```python
from build123d import *

# Parameters (mm, degrees)
SKETCH1_W           = 50.8
SKETCH1_H           = 61.92
BOSS_EXTRUDE2_DEPTH = 3.175
SKETCH2_R           = 12.5
SKETCH2_R_2         = 2.75
CUT_EXTRUDE1_DEPTH  = 4.175


with BuildPart() as part:
    # Sketch1 → Boss-Extrude2 (new body)
    with BuildSketch(Plane(origin=(0, 0, 0), x_dir=(0, 0, -1), z_dir=(1, 0, 0))):
        with Locations((25.4, 30.96)):
            Rectangle(SKETCH1_W, SKETCH1_H)
    extrude(amount=BOSS_EXTRUDE2_DEPTH)

    # Sketch2 → Cut-Extrude1 (cut, through all)
    with BuildSketch(Plane.ZY):
        with Locations((-25.399655405, 30.96)):
            Circle(SKETCH2_R)
        with Locations((-43.35992398, 48.920755906)):
            Circle(SKETCH2_R_2)
        with Locations((-25.399655405, 56.36)):
            Circle(SKETCH2_R_2)
        with Locations((-5.004504526, 56.648087135)):
            Circle(SKETCH2_R_2)
        with Locations((-25.399655405, 5.560695)):
            Circle(SKETCH2_R_2)
        with Locations((-45.795509398, 5.272471121)):
            Circle(SKETCH2_R_2)
        with Locations((-7.439487758, 13.000182758)):
            Circle(SKETCH2_R_2)
    extrude(amount=-CUT_EXTRUDE1_DEPTH, mode=Mode.SUBTRACT)


solid = part.part
```
Could you check a few things on this model? Use its own coordinates, in mm. Coordinates: 2 decimals unless noted, no trailing zeros. Write each loop counter-clockwise with the first axis right and the second up, starting at its lowest first coordinate (ties: lowest second). Pieces come first, ordered by that corner, then holes. Notation, with made-up numbers: (-12.75, 89.25) -> (26.25, 89.25) arc R16 ccw to (26.25, 94.25) -> close; hole circle Ø8 at (-33, 28.25). An arc over 180 degrees is marked (long way). Write item = value, one per line. Start each with the question number.
(1) I want a section at B-B (z = -32.5). Please give me the cut outline in (x, y) (3 decimals), plus the area to 3 significant figures.
(2) I want a section at C-C (z = -45). Please give me the cut outline in (x, y) (3 decimals), plus the area to 3 significant figures.
(3) I want a section at A-A (y = 30.96). Please give me the cut outline in (x, z) (3 decimals), plus the area to 3 significant figures.
(4) We'd pull the mould along Y, two halves only. Please class faces 1 (the face through (2, 31, -50.8)), 2 (the face through (1.565, 59.375, -5.362)), 3 (the face through (2, 61.92, -25)): released by +Y, released by -Y, zero draft, split by the parting line, or undercut.
(5) I want a section at D-D (x = 1.65). Please give me the cut outline in (y, z), plus the area to 3 significant figures.
(6) Will this pin go through, and if not, where does the flat tip stop? pin 1 (1 mm diameter, centred on x = 0.5, z = -31.5, fed in from -Y).
(7) I need wall thicknesses on line 1 (Z direction, x = 0.4, y = 5.5); line 2 (Z direction, x = 1.55, y = 13); line 3 (Z direction, x = 1.6, y = 31). Which ranges of each line are inside material? Lowest first, please. Write a range as [from, to].
Result set:
q1.outline = (0, 0) -> (3.175, 0) -> (3.175, 20.672) -> (0, 20.672) -> close; (0, 41.248) -> (3.175, 41.248) -> (3.175, 61.92) -> (0, 61.92) -> close
q1.area = 131 mm2
q2.outline = (0, 0) -> (3.175, 0) -> (3.175, 2.64) -> (0, 2.64) -> close; (0, 7.905) -> (3.175, 7.905) -> (3.175, 46.713) -> (0, 46.713) -> close; (0, 51.128) -> (3.175, 51.128) -> (3.175, 61.92) -> (0, 61.92) -> close
q2.area = 166 mm2
q3.outline = (0, -50.8) -> (3.175, -50.8) -> (3.175, -37.9) -> (0, -37.9) -> close; (0, -12.9) -> (3.175, -12.9) -> (3.175, 0) -> (0, 0) -> close
q3.area = 81.9 mm2
q4.face_1 = zero draft
q4.face_2 = undercut
q4.face_3 = released by +Y
q5.outline = (0, -50.8) -> (61.92, -50.8) -> (61.92, 0) -> (0, 0) -> close; hole circle Ø5.5 at (5.27, -45.8); hole circle Ø5.5 at (5.56, -25.4); hole circle Ø5.5 at (13, -7.44); hole circle Ø25 at (30.96, -25.4); hole circle Ø5.5 at (48.92, -43.36); hole circle Ø5.5 at (56.36, -25.4); hole circle Ø5.5 at (56.65, -5)
q5.area = 2,510 mm2
q6.pin_1 = 0
q7.line_1 = [-50.8, -48.54], [-43.05, -28.15], [-22.65, 0]
q7.line_2 = [-50.8, -10.19], [-4.69, 0]
q7.line_3 = [-50.8, -37.9], [-12.9, 0]
